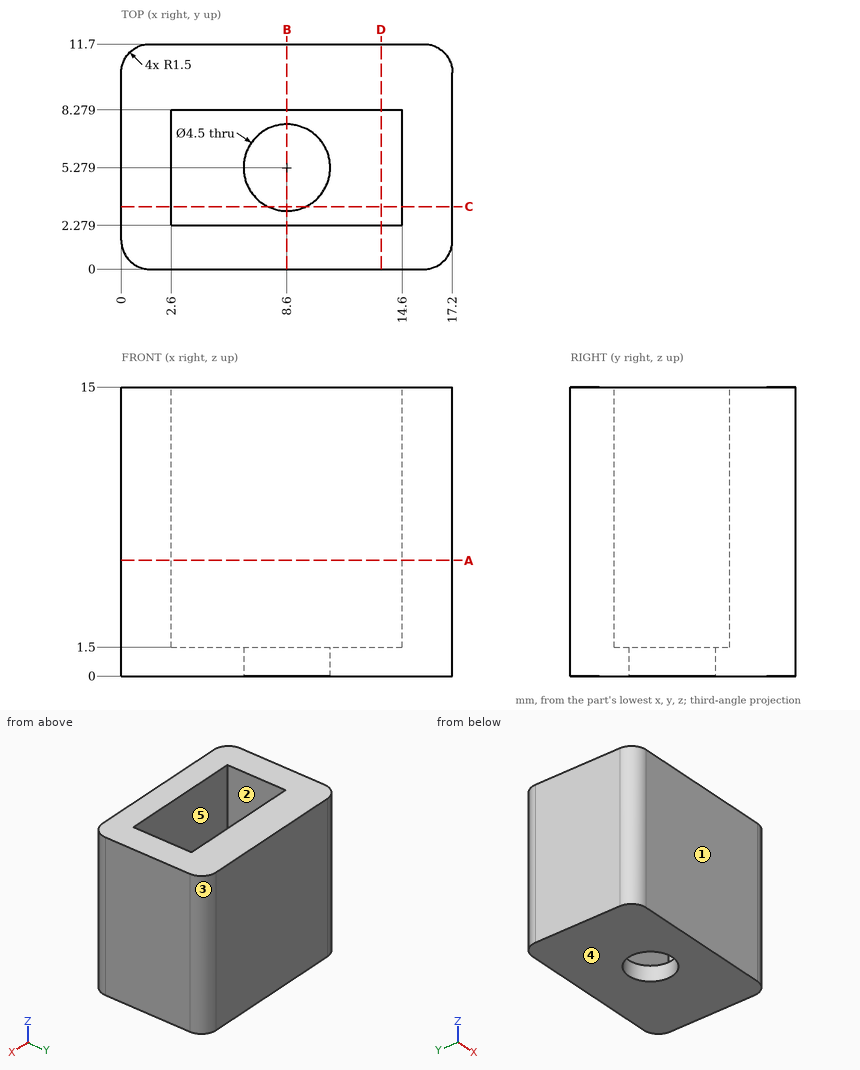
For this review, use the dimensioned drawing (mm, ordinates from the lowest corner) and the shaded views. A direction names the side the tool comes from. Give positions to 0.01 mm unless a question says otherwise; leave off trailing zeros. Order: outer loops, then holes, each group sorted by start corner. A loop starts at its lowest first (then second) coordinate and runs counter-clockwise, first axis right, second up.
1. For pin 1 Ø6 at (y, z) = (7, 3.5) entering from -X, flat-tipped, find the tip position at first contact; note if it passes through.
Solution:
pin 1: stops at x = 0
2. Add section D-D, the plane x = 13.5. State the section outline as (y, z) points.
Solution:
outline: (0, 0) - (11.7, 0) - (11.7, 15) - (8.28, 15) - (8.28, 1.5) - (2.28, 1.5) - (2.28, 15) - (0, 15) - close
3. Add section B-B, the plane x = 8.6. State the section outline as (y, z) points.
Solution:
outline: (0, 0) - (3.03, 0) - (3.03, 1.5) - (2.28, 1.5) - (2.28, 15) - (0, 15) - close; (7.53, 0) - (11.7, 0) - (11.7, 15) - (8.28, 15) - (8.28, 1.5) - (7.53, 1.5) - close
4. Mouldability with a two-part tool opening along Y and no side actions: class the marked faces 3, 4 and 5 as +Y half, -Y half, draft (parallel to the pull), parting line (faces both ways), or undercut.
Solution:
face 3: +Y half
face 4: draft
face 5: undercut
5. Add section C-C, the plane y = 3.25. State the section outline as (x, z) points.
Solution:
outline: (0, 0) - (7.63, 0) - (7.63, 1.5) - (2.6, 1.5) - (2.6, 15) - (0, 15) - close; (9.57, 0) - (17.2, 0) - (17.2, 15) - (14.6, 15) - (14.6, 1.5) - (9.57, 1.5) - close
6. To check wall thickness, follow L1, parallel to Y at x = 13.25, z = 8.5; L2, parallel to Y at x = 8.6, z = 1.1; L3, parallel to X at y = 6.75, z = 10. State the ranges of each line that lie inside material, in increasing order.
Solution:
L1: y = 0 to 2.28, 8.28 to 11.7
L2: y = 0 to 3.03, 7.53 to 11.7
L3: x = 0 to 2.6, 14.6 to 17.2
7. Tool access review of the marked faces 1 and 2: name each direction out of +Z, -Z, +X, -X, +Y, -Y from which nothing blocks a thin tool from reaching the whole face with its end or side.
Solution:
face 1: +Z, -Z, +X, -X, -Y
face 2: +Z
8. Add section A-A, the plane z = 6. State the section outline as (x, y) points, then the cut area to 3 significant figures.
Solution:
outline: (0, 1.5) arc R1.5 ccw to (1.5, 0) - (15.7, 0) arc R1.5 ccw to (17.2, 1.5) - (17.2, 10.2) arc R1.5 ccw to (15.7, 11.7) - (1.5, 11.7) arc R1.5 ccw to (0, 10.2) - close; hole (2.6, 2.28) - (14.6, 2.28) - (14.6, 8.28) - (2.6, 8.28) - close
area: 127 mm2
